Here's the drawing with two shaded views (mm, measured from the low corner). I have some questions. Give positions to 0.01 mm unless a question says otherwise; leave off trailing zeros. Loops run counter-clockwise (first coordinate to the right, second up) from the corner with the lowest first, then second, coordinate; pieces in that order, holes last. Notation, with made-up numbers: (26.25, 80) - (56.25, 80) arc R23 ccw to (56.25, 92) - close; hole circle Ø4 at (-21.75, 55). An arc over 180 degrees is marked (long way). Write each question's results on one line, items separated by ' | '. Start each with the question number.
1) If I drill on probe 1 along Y at (x, z) = (1.75, 0.8); probe 2 along X at (y, z) = (2.8, 0.4); probe 3 along X at (y, z) = (2.5, 0.15) (1 decimal), over which ranges is the centre line in solid material (lowest first)? Write a range as [from, to].
2) If we mould it in two halves opening along X, with no side actions, what happens to the marked faces 1, 2 and 3? For each: +X half, -X half, draft (parallel to the pull), parting line (faces both ways), or undercut.
3) I want a section at C-C, the plane z = 0.55. Write out the boundary of the cut face in (x, y).
4) I want a section at B-B, the plane y = 2. Write out the boundary of the cut face in (x, z).
5) I want a section at A-A, the plane x = 6.2. Write out the boundary of the cut face in (y, z).
6) I want a section at D-D, the plane x = 1. Write out the boundary of the cut face in (y, z).
7) I'm going to push flat-ended pins straight in: pin 1 (1 mm diameter, centred on x = 7, y = 3, fed in from -Z); pin 2 (1.4 mm diameter, centred on x = 1.8, y = 2, fed in from -Z). Where does each tip first touch, or does it pass through?
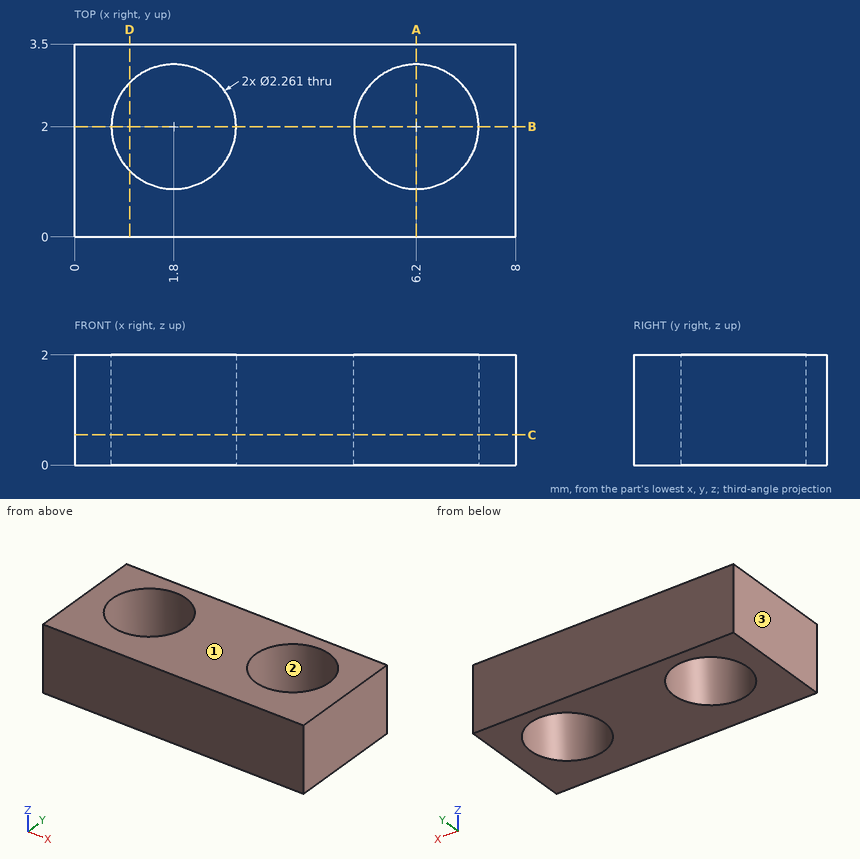
Answers:
1) probe 1: y = [0, 0.87], [3.13, 3.5] | probe 2: x = [0, 1], [2.6, 5.4], [7, 8] | probe 3: x = [0, 0.8], [2.8, 5.2], [7.2, 8]
2) face 1: draft | face 2: undercut | face 3: -X half
3) outline: (0, 0) - (8, 0) - (8, 3.5) - (0, 3.5) - close; hole circle Ø2.26 at (1.8, 2); hole circle Ø2.26 at (6.2, 2)
4) outline: (0, 0) - (0.67, 0) - (0.67, 2) - (0, 2) - close; (2.93, 0) - (5.07, 0) - (5.07, 2) - (2.93, 2) - close; (7.33, 0) - (8, 0) - (8, 2) - (7.33, 2) - close
5) outline: (0, 0) - (0.87, 0) - (0.87, 2) - (0, 2) - close; (3.13, 0) - (3.5, 0) - (3.5, 2) - (3.13, 2) - close
6) outline: (0, 0) - (1.2, 0) - (1.2, 2) - (0, 2) - close; (2.8, 0) - (3.5, 0) - (3.5, 2) - (2.8, 2) - close
7) pin 1: stops at z = 0 | pin 2: passes through
